```python
from build123d import *

# Parameters (mm, degrees)
F1_DEPTH = 6.35
F2_R     = 5.08
F3_SIZE  = 5.08


with BuildPart() as f1:
    # F0 (on Front) → F1 (new body, symmetric)
    with BuildSketch(Plane.XZ):
        Polygon((11.43, -54.61), (11.43, 54.61), (3.81, 54.61), (3.81, 6.35), (-3.81, 6.35), (-3.81, 54.61), (-11.43, 54.61), (-11.43, -54.61), (-3.81, -54.61), (-3.81, -6.35), (3.81, -6.35), (3.81, -54.61), align=None)
    extrude(amount=F1_DEPTH, both=True)

    # F2
    f2_edges = [f1.edges().sort_by_distance(p)[0] for p in [
        (-3.81, 0, 54.61),
        (3.81, 0, 54.61),
    ]]
    fillet(f2_edges, radius=F2_R)

    # F3
    f3_edges = [f1.edges().sort_by_distance(p)[0] for p in [
        (-11.43, 0, -54.61),
        (11.43, 0, -54.61),
    ]]
    chamfer(f3_edges, length=F3_SIZE)


solid = f1.part
```
For this review, take the finished solid that the model builds, in its own axes (mm). A direction names the side the tool comes from. Round coordinates to 2 decimals unless told otherwise and drop trailing zeros. Write each loop counter-clockwise with the first axis right and the second up, starting at its lowest first coordinate (ties: lowest second). Pieces come first, ordered by that corner, then holes. Notation, with made-up numbers: (17.25, -26) - (56.25, -26) arc R27 ccw to (56.25, 13) - close; hole circle Ø5 at (-15, -15.75). An arc over 180 degrees is marked (long way). Answer as CSV lines item,"result". Start each with the question number.
(1) Machinability: for faces 4 (the cylindrical face through (5.259, -0.089, 53.082)), 5 (the flat face through (-10, 0, 54.61)), 6 (the flat face through (0, 0, -6.35)), which of the approach directions +Z, -Z, +X, -X, +Y, -Y give a long, thin tool a straight path to every point of the face, cutting with its end or side? Answer none if there is none.
(2) For pin 1 (2 mm diameter, centred on x = -3.5, y = -2, fed in from -Z); pin 2 (6 mm diameter, centred on x = -0.5, y = -3, fed in from +Z); pin 3 (2.5 mm diameter, centred on x = 0.5, y = -0.5, fed in from -Z), all flat-tipped, find the tip position at first contact; note any pin that passes through.
(3) Mouldability with a two-part tool opening along X and no side actions: class faces 1 (the cylindrical face through (-5.338, -0.089, 53.161)), 2 (the flat face through (0, -6.35, 1)), 3 (the flat face through (8.85, -0.09, -52.11)) as +X half, -X half, draft (parallel to the pull), parting line (faces both ways), or undercut.
(4) For line 1 (X direction, y = 5, z = 22); line 2 (Z direction, x = -3.5, y = 0.5); line 3 (Z direction, x = -5.5, y = -4.5), list the stretches that pass through material, from the lowest coordinate up.
(5) Add section C-C, the plane x = -1.25. State the section outline as (y, z) points.
(6) Add section B-B, the plane y = 0.25. State the section outline as (x, z) points, plus the area to 3 significant figures.
(7) Add section A-A, the plane z = -39. State the section outline as (x, y) points.
From the geometry:
1,face 4,"+Z, +Y, -Y"
1,face 5,"+Z, +X, -X, +Y, -Y"
1,face 6,"-Z, +Y, -Y"
2,pin 1,"stops at z = -54.61"
2,pin 2,"stops at z = 6.35"
2,pin 3,"stops at z = -6.35"
3,face 1,"undercut"
3,face 2,"draft"
3,face 3,"+X half"
4,line 1,"x = -11.43 to -3.81, 3.81 to 11.43"
4,line 2,"z = -6.35 to 6.35"
4,line 3,"z = -54.61 to 53.31"
5,outline,"(-6.35, -6.35) - (6.35, -6.35) - (6.35, 6.35) - (-6.35, 6.35) - close"
6,outline,"(-11.43, -49.53) - (-6.35, -54.61) - (-3.81, -54.61) - (-3.81, -6.35) - (3.81, -6.35) - (3.81, -54.61) - (6.35, -54.61) - (11.43, -49.53) - (11.43, 54.61) - (8.89, 54.61) arc R5.08 ccw to (3.81, 49.53) - (3.81, 6.35) - (-3.81, 6.35) - (-3.81, 49.53) arc R5.08 ccw to (-8.89, 54.61) - (-11.43, 54.61) - close"
6,area,"1,720 mm²"
7,outline,"(-11.43, -6.35) - (-3.81, -6.35) - (-3.81, 6.35) - (-11.43, 6.35) - close; (3.81, -6.35) - (11.43, -6.35) - (11.43, 6.35) - (3.81, 6.35) - close"
